Check sheet for the modelled part. Datum: model origin and axes. Units: mm. Face numbers are marked on the shaded views. Give positions to 0.01 mm unless a question says otherwise; leave off trailing zeros. Loops run counter-clockwise (first coordinate to the right, second up) from the corner with the lowest first, then second, coordinate; pieces in that order, holes last. Notation, with made-up numbers: M 29,78 L 46,78 A30 cw 46,108 Z; hole C -32.75,-32.75 d10. An arc over 180 degrees is marked long. Put each result on its own line as item: value. Start each with the question number.
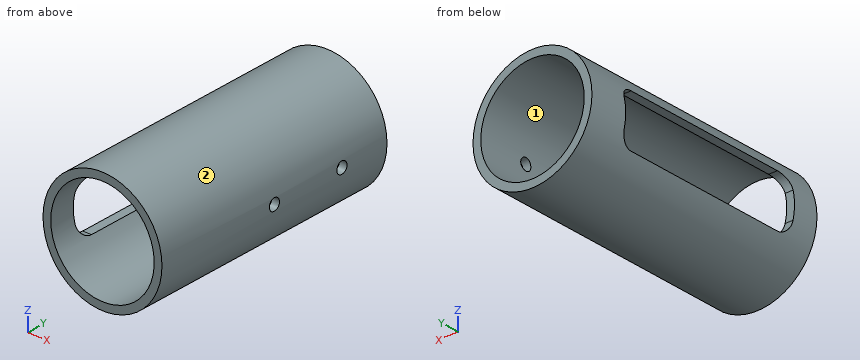
Autodesk Inventor part; units mm, degrees
ref_plane "YZ Plane" through (0, 0, 0) normal (1, 0, 0) x (0, 1, 0)
ref_plane "XZ Plane" through (0, 0, 0) normal (0, 1, 0) x (-1, 0, 0)
ref_plane "XY Plane" through (0, 0, 0) normal (0, 0, 1) x (1, 0, 0)
sketch "Sketch1" plane through (0, 0, 0) normal (0, 1, 0) x (-1, 0, 0)
  circle A0 centre (0, 0) radius 23
  circle A1 centre (0, 0) radius 20
  dimension "d0" = 3
  dimension "d1" = 40
extrude "Extrusion1" add sketch "Sketch1" along normal blind 100
sketch "Sketch2" plane through (0, 0, 0) normal (0, 0, 1) x (1, 0, 0)
  line L0 (-23, 85) -> (0, 85)
  line L1 (0, 85) -> (0, 10)
  line L2 (0, 10) -> (-23, 10)
  line L3 (-23, 10) -> (-23, 85)
  line L4 (23, 100) -> (-23, 100)
  line L5 (-23, 0) -> (23, 0)
  point P0 (0, 0)
  dimension "d4" = 75
  dimension "d5" = 10
extrude "Extrusion2" cut sketch "Sketch2" along normal mid plane 20
fillet "Fillet1" radius 5 4 edges at (-19.0164, 85, -10) (-19.0164, 85, 10) (-19.0164, 10, 10) (-19.0164, 10, -10)
sketch "Sketch3" plane through (0, 0, 0) normal (1, 0, 0) x (0, 1, 0)
  line L0 (-20, 0) -> (120, 0)
  line L1 (85, -5) -> (85, 5)
  line L2 (100, 20) -> (100, -20)
  point P0 (0, 0)
  point P1 (80, 0)
  point P2 (50, 0)
  dimension "d9" = 30
  dimension "d18" = 20
hole "Hole1" at (0, 80, 0) at (0, 50, 0) direction (1, 0, 0) diameter 4.5 end through all
properties part number "Pancake_PVC Pipe" material "PVC-Piping"
Q1. Depth check by flat-ended pin: P1, Ø6, axis at x = 14, y = 31.5, coming from the +Z side; P2, Ø3, axis at x = 0.5, y = 27, coming from the -Z side; P3, Ø1, axis at x = -19.5, y = 35, coming from the +Z side. Enter the tip coordinate at first touch or a pass-through.
Q2. Section check B-B, the plane x = 0. Record the cut outline in (y, z).
Q3. Section check D-D, the plane y = 50. Record the cut outline in (x, z).
Q4. Section check A-A, the plane z = 0. Record the cut outline in (x, y), then the cut area to 3 significant figures.
Q5. Section check C-C, the plane z = -7. Record the cut outline in (x, y) (3 decimals).
Q6. Mould release check, pull along X, two halves, no side actions. Record for the marked faces 1 and 2: pulls with the +X half, pulls with the -X half, needs draft (parallel to the pull), parting line crosses it, or undercut.
Q7. Thickness scan on line 1 along Z through (x, y) = (0, 35); line 2 along X through (y, z) = (54.5, -0.5); line 3 along Z through (x, y) = (9, 16). Record the ranges inside material, lowest first. Write a range as [from, to].
Found:
1. P1: stops at z = 20.2
1. P2: stops at z = -23
1. P3: stops at z = 12.96
2. outline: M 0,-23 L 100,-23 L 100,-20 L 0,-20 Z; M 0,20 L 100,20 L 100,23 L 0,23 Z
3. outline: M -20.71,-10 A23 ccw 22.89,-2.25 L 19.87,-2.25 A20 cw -17.32,-10 Z; M -20.71,10 L -17.32,10 A20 cw 19.87,2.25 L 22.89,2.25 A23 ccw Z
4. outline: M -23,0 L -20,0 L -20,10 L -23,10 Z; M -23,85 L -20,85 L -20,100 L -23,100 Z; M 20,0 L 23,0 L 23,47.75 L 20,47.75 Z; M 20,52.25 L 23,52.25 L 23,77.75 L 20,77.75 Z; M 20,82.25 L 23,82.25 L 23,100 L 20,100 Z
4. area: 348 mm^2
5. outline: M -21.909,0 L -18.735,0 L -18.735,10.417 L -21.909,10.417 Z; M -21.909,84.583 L -18.735,84.583 L -18.735,100 L -21.909,100 Z; M 18.735,0 L 21.909,0 L 21.909,100 L 18.735,100 Z
6. face 1: undercut
6. face 2: parting line crosses it
7. line 1: z = [-23, -20], [20, 23]
7. line 2: x = [19.99, 22.99]
7. line 3: z = [-21.17, -17.86], [17.86, 21.17]
